For this review, take the finished solid that the model builds, in its own axes (mm). A direction names the side the tool comes from. Coordinates: 2 decimals unless noted, no trailing zeros. Loops run counter-clockwise (first coordinate to the right, second up) from the corner with the lowest first, then second, coordinate; pieces in that order, holes last.
1. To check wall thickness, follow probe 1 along X at (y, z) = (9.5, 2.5) (3 decimals); probe 2 along Z at (x, y) = (33.5, 1); probe 3 along X at (y, z) = (-16, 3.25). State the ranges of each line that lie inside material, in increasing order.
2. Take a section at B-B, the plane y = -2. State the section outline as (x, z) points (3 decimals), then the cut area to 3 significant figures.
3. Take a section at C-C, the plane z = 1.5. State the section outline as (x, y) points (1 decimal), then the cut area to 3 significant figures.
4. Mouldability with a two-part tool opening along Y and no side actions: class faces 4 (the face through (-29.121, 7, 1)), 5 (the face through (46.901, 16.143, 1.288)), 6 (the face through (42.858, 7.839, 1.252)) as pulls with the +Y half, pulls with the -Y half, needs draft (parallel to the pull), parting line crosses it, or undercut.
5. Machinability: for faces 1 (the face through (-29.845, 16.143, 1.288)), 2 (the face through (-41.52, -9.15, 4.73)), 3 (the face through (0.6, 4.57, 4.67)), which of the approach directions +Z, -Z, +X, -X, +Y, -Y give a long, thin tool a straight path to every point of the face, cutting with its end or side? Answer none if there is none.
6. Clearance check with flat-ended pins moving along their axes: P1, Ø1.5, axis at x = -24, z = 6, coming from the +Y side; P2, Ø2, axis at x = 37.5, z = 2, coming from the -Y side; P3, Ø1.5, axis at x = -27.5, y = 3, coming from the -Z side; P4, Ø1.5, axis at x = -26, z = 2, coming from the -Y side. State where each tip first meets the part, or that it passes through.
7. Take a section at A-A, the plane x = -38.1. State the section outline as (y, z) points, then the cut area to 3 significant figures.
8. Take a section at D-D, the plane x = -6. State the section outline as (y, z) points, then the cut area to 3 significant figures.
```python
from build123d import *

# Parameters (mm, degrees)
SKETCH1_R           = 4.762500000000004
BOSS_EXTRUDE1_DEPTH = 2.54
BOSS_EXTRUDE2_DEPTH = 4.318
FILLET1_R           = 2.54


with BuildPart() as part:
    # Sketch1 → Boss-Extrude1 (new body)
    with BuildSketch(Plane.XY):
        with BuildLine():
            Line((-29.12070870680529, -1.1283392484503774), (-29.12070870680529, 16.90683065104644))
            Line((-29.12070870680529, 16.90683065104644), (-47.625, 16.906830651046437))
            Line((-47.625, 16.906830651046437), (-47.625, -6.402026683274578))
            Line((-47.625, -6.402026683274578), (-24.11489201542563, -22.209169348953562))
            ThreePointArc((-24.11489201542563, -22.209169348953562), (4.67e-15, -18.29272199465825), (24.11489201542563, -22.209169348953562))
            Line((24.11489201542563, -22.209169348953562), (47.625, -6.402026683274578))
            Line((47.625, -6.402026683274578), (47.625, 16.906830651046437))
            Line((47.625, 16.906830651046437), (29.12070870680529, 16.90683065104644))
            Line((29.12070870680529, 16.90683065104644), (29.12070870680529, -1.1283392484503774))
            ThreePointArc((29.12070870680529, -1.1283392484503774), (4.67e-15, 4.6555807384347645), (-29.12070870680529, -1.1283392484503774))
        make_face()
        with Locations((-38.099999999999994, 8.048015683552894)):
            Circle(SKETCH1_R, mode=Mode.SUBTRACT)
        with Locations(Location((38.099999999999994, 8.048015683552894, 0), (0, 0, 180))):
            Circle(SKETCH1_R, mode=Mode.SUBTRACT)
    extrude(amount=BOSS_EXTRUDE1_DEPTH)

    # Sketch2 → Boss-Extrude2 (add)
    with BuildSketch(Plane.XY.offset(2.54)):
        with BuildLine():
            Line((-43.56033013161569, -9.13492848621798), (-24.114892015425625, -22.209169348953562))
            ThreePointArc((-24.114892015425625, -22.209169348953562), (4.67e-15, -18.29272199465825), (24.11489201542563, -22.209169348953562))
            Line((24.11489201542563, -22.209169348953562), (43.58710776229448, -9.11692440777367))
            ThreePointArc((43.58710776229448, -9.11692440777367), (0.01055892070138382, 4.5719736134911955), (-43.56033013161569, -9.13492848621798))
        make_face()
    extrude(amount=BOSS_EXTRUDE2_DEPTH)

    # Fillet1
    fillet1_edges = [part.edges().sort_by_distance(p)[0] for p in [
        (47.625, -6.402026683274578, 1.27),
        (-47.625, -6.402026683274578, 1.27),
        (-47.625, 16.906830651046437, 1.27),
        (-29.12070870680529, 16.90683065104644, 1.27),
        (29.12070870680529, 16.90683065104644, 1.27),
        (47.625, 16.906830651046437, 1.27),
        (43.58710776229448, -9.116924407773672, 4.699),
        (-43.56033013161569, -9.13492848621799, 4.699),
    ]]
    fillet(fillet1_edges, radius=FILLET1_R)


solid = part.part
```
Results list:
1. probe 1: x = -47.625 to -42.636, -33.564 to -29.121, 29.121 to 33.564, 42.636 to 47.625
1. probe 2: z = 0 to 2.54
1. probe 3: x = -33.35 to 33.35
2. outline: (-47.625, 0) - (47.625, 0) - (47.625, 2.54) - (30.974, 2.54) - (30.974, 6.858) - (-30.922, 6.858) - (-30.922, 2.54) - (-47.625, 2.54) - close
2. area: 509 mm2
3. outline: (-47.6, -5) arc R2.5 ccw to (-46.5, -7.2) - (-24.1, -22.2) arc R76.2 cw to (24.1, -22.2) - (46.5, -7.2) arc R2.5 ccw to (47.6, -5) - (47.6, 14.4) arc R2.5 ccw to (45.1, 16.9) - (31.7, 16.9) arc R2.5 ccw to (29.1, 14.4) - (29.1, -1.1) arc R76.2 ccw to (-29.1, -1.1) - (-29.1, 14.4) arc R2.5 ccw to (-31.7, 16.9) - (-45.1, 16.9) arc R2.5 ccw to (-47.6, 14.4) - close; hole circle Ø9.5 at (-38.1, 8); hole circle Ø9.5 at (38.1, 8)
3. area: 2,250 mm2
4. face 4: needs draft
4. face 5: pulls with the +Y half
4. face 6: undercut
5. face 1: +Z, -Z, +Y
5. face 2: +Z, -X
5. face 3: +Z, +Y
6. P1: stops at y = 0.93
6. P2: stops at y = -13.88
6. P3: passes through
6. P4: stops at y = -21.45
7. outline: (-12.81, 0) - (3.29, 0) - (3.29, 2.54) - (-5.66, 2.54) - (-5.66, 6.86) - (-12.81, 6.86) - close; (12.81, 0) - (16.91, 0) - (16.91, 2.54) - (12.81, 2.54) - close
7. area: 82.1 mm2
8. outline: (-18.53, 0) - (4.42, 0) - (4.42, 2.54) - (4.33, 2.54) - (4.33, 6.86) - (-18.53, 6.86) - close
8. area: 157 mm2
